Build history of the part. All positions in model axes, mm. A direction names the side the tool comes from. Coordinates: 2 decimals unless noted, no trailing zeros. Loops run counter-clockwise (first coordinate to the right, second up) from the corner with the lowest first, then second, coordinate; pieces in that order, holes last.
(1) Wall check: L1, parallel to Y at x = 0, z = -0.7; L2, parallel to X at y = -41, z = 12; L3, parallel to Y at x = -8.5, z = 7.25. Give the ranges that are in metal, low to high.
(2) Slice it at B-B (x = 0). Give the number of separate pieces and of enclosed holes in the cut face, and give its area (4 significant figures).
(3) Flat gauge pins, fed straight in: P1, Ø2, axis at x = 30.5, z = 4, coming from the +Y side; P2, Ø5, axis at x = -1, y = -35.5, coming from the +Z side; P3, Ø0.5, axis at x = -31, z = 19, coming from the -Y side. Where does each tip first touch, or does it go through?
(4) Slice it at A-A (z = 13). Give the cut face in (x, y).
(5) Tool access for faces 4 (the face through (-27, 16, 6)), 5 (the face through (28, 43.5, 17)), 6 (the face through (-29, 16, 11)): list every direction of +Z, -Z, +X, -X, +Y, -Y with a clear straight run to the whole face (end or side of a thin tool).
(6) Slice it at D-D (x = -9). Give the cut face in (y, z).
(7) Two-plate mould, pull along Y, no slides. Class faces 1 (the face through (31.297, 48.859, 8.633)), 2 (the face through (-32.5, -1, 9)), 3 (the face through (-30, 41.5, 9)): pulls with the +Y half, pulls with the -Y half, needs draft (parallel to the pull), parting line crosses it, or undercut.
from build123d import *

# Parameters (mm, degrees)
SKETCH_1_W            = 65
SKETCH_1_H            = 100
SKETCH_1_W_2          = 63
SKETCH_1_H_2          = 98
EXTRUDE_1_DEPTH       = 18
SKETCH_3_W            = 65
SKETCH_3_H            = 100
EXTRUDE_2_DEPTH       = 1
SKETCH_4_W            = 7.5
SKETCH_4_H            = 7
SKETCH_4_H_2          = 8
EXTRUDE_3_DEPTH       = 11
SKETCH_8_W            = 7.5
SKETCH_8_H            = 7.5
EXTRUDE_4_DEPTH       = 18
EXTRUDE_10_DEPTH      = 1.5
EXTRUDE_10_DEPTH_BACK = 1.5
SKETCH_17_W           = 48
SKETCH_17_H           = 1
SKETCH_17_W_2         = 1
SKETCH_17_H_2         = 83
SKETCH_11_R           = 3
CUT_EXTRUDE_2_DEPTH   = 18
HOLE_WIZARD_M31_D     = 3.4
SKETCH_5_R            = 1.3
CUT_EXTRUDE_4_DEPTH   = 5
SKETCH_15_W           = 4
SKETCH_15_H           = 10
CUT_EXTRUDE_3_DEPTH   = 1
FILLET_5_R            = 1.5
FILLET_6_R            = 3.5
FILLET_7_R            = 4
SKETCH_16_R           = 6
SKETCH_16_R_2         = 5
EXTRUDE_6_DEPTH       = 2
SKETCH_10_6_R         = 3
SKETCH_10_6_R_2       = 2.5
EXTRUDE_8_DEPTH       = 5
SKETCH_9_4_R          = 4
SKETCH_9_4_R_2        = 2.5
SKETCH_9_4_R_3        = 3
CUT_EXTRUDE_6_DEPTH   = 63.741533293
FILLET_8_R            = 4


with BuildPart() as part:
    # Эскиз1 → Бобышка-Вытянуть1 (new body)
    with BuildSketch(Plane.XY):
        Rectangle(SKETCH_1_W, SKETCH_1_H)
        Rectangle(SKETCH_1_W_2, SKETCH_1_H_2, mode=Mode.SUBTRACT)
    extrude(amount=EXTRUDE_1_DEPTH)

    # Эскиз3 → Бобышка-Вытянуть2 (add)
    with BuildSketch(Plane(origin=(0, 0, 0), x_dir=(-1, 0, 0), z_dir=(0, 0, -1))):
        Rectangle(SKETCH_3_W, SKETCH_3_H)
    extrude(amount=EXTRUDE_2_DEPTH)

    # Эскиз4 → Бобышка-Вытянуть3 (add)
    with BuildSketch(Plane.XY):
        with Locations((-27.75, 16)):
            Rectangle(SKETCH_4_W, SKETCH_4_H)
        with Locations((27.75, 16)):
            Rectangle(SKETCH_4_W, SKETCH_4_H)
        with Locations((-27.75, -37.5)):
            Rectangle(SKETCH_4_W, SKETCH_4_H_2)
        with Locations((27.75, -37.5)):
            Rectangle(SKETCH_4_W, SKETCH_4_H_2)
    extrude(amount=EXTRUDE_3_DEPTH)

    # Эскиз8 → Бобышка-Вытянуть4 (add)
    with BuildSketch(Plane.XY):
        with Locations((-27.75, 45.25)):
            Rectangle(SKETCH_8_W, SKETCH_8_H)
        with Locations((27.75, 45.25)):
            Rectangle(SKETCH_8_W, SKETCH_8_H)
        with Locations((27.75, -45.25)):
            Rectangle(SKETCH_8_W, SKETCH_8_H)
        with Locations((-27.75, -45.25)):
            Rectangle(SKETCH_8_W, SKETCH_8_H)
    extrude(amount=EXTRUDE_4_DEPTH)

    # Эскиз17 → Бобышка-Вытянуть10 (add, two sides: drawn at the far end of the back side and taken through both)
    with BuildSketch(Plane.XY.offset(18).offset(-EXTRUDE_10_DEPTH_BACK)):
        with Locations((0, 48.5)):
            Rectangle(SKETCH_17_W, SKETCH_17_H)
        with Locations((31, 0)):
            Rectangle(SKETCH_17_W_2, SKETCH_17_H_2)
        with Locations((-31, 0)):
            Rectangle(SKETCH_17_W_2, SKETCH_17_H_2)
        with Locations((0, -48.5)):
            Rectangle(SKETCH_17_W, SKETCH_17_H)
    extrude(amount=EXTRUDE_10_DEPTH + EXTRUDE_10_DEPTH_BACK)

    # Эскиз11 → Вырез-Вытянуть2 (cut)
    with BuildSketch(Plane(origin=(0, 0, -1), x_dir=(-1, 0, 0), z_dir=(0, 0, -1))):
        with Locations((-28, 45.5)):
            Circle(SKETCH_11_R)
        with Locations((28, 45.5)):
            Circle(SKETCH_11_R)
        with Locations((28, -45.5)):
            Circle(SKETCH_11_R)
        with Locations((-28, -45.5)):
            Circle(SKETCH_11_R)
    extrude(amount=-CUT_EXTRUDE_2_DEPTH, mode=Mode.SUBTRACT)

    # Отверстие с зазором M31 (through all)
    with Locations(Plane(origin=(0, 0, 17), x_dir=(-1, 0, 0), z_dir=(0, 0, -1))):
        with Locations((-28, 45.5), (28, 45.5), (28, -45.5), (-28, -45.5)):
            Hole(HOLE_WIZARD_M31_D / 2)

    # Эскиз5 → Вырез-Вытянуть4 (cut)
    with BuildSketch(Plane.XY.offset(11)):
        with Locations((-27, 16)):
            Circle(SKETCH_5_R)
        with Locations((27, 16)):
            Circle(SKETCH_5_R)
        with Locations((-27, -37)):
            Circle(SKETCH_5_R)
        with Locations((27, -37)):
            Circle(SKETCH_5_R)
    extrude(amount=-CUT_EXTRUDE_4_DEPTH, mode=Mode.SUBTRACT)

    # Эскиз15 → Вырез-Вытянуть3 (cut)
    with BuildSketch(Plane.ZY.offset(31.5)):
        with Locations((9.4, -23.5)):
            Rectangle(SKETCH_15_W, SKETCH_15_H)
    extrude(amount=CUT_EXTRUDE_3_DEPTH, mode=Mode.SUBTRACT)

    # Скругление5
    fillet_5_edges = [part.edges().sort_by_distance(p)[0] for p in [
        (-32, -18.5, 11.4),
        (-32, -28.5, 11.4),
        (-32, -28.5, 7.4),
        (-32, -18.5, 7.4),
    ]]
    fillet(fillet_5_edges, radius=FILLET_5_R)

    # Скругление6
    fillet_6_edges = [part.edges().sort_by_distance(p)[0] for p in [
        (-24, 12.5, 5.5),
        (-24, 19.5, 5.5),
        (24, 19.5, 5.5),
        (24, 12.5, 5.5),
        (-24, -33.5, 5.5),
        (24, -33.5, 5.5),
    ]]
    fillet(fillet_6_edges, radius=FILLET_6_R - 0.0001)  # a hair under: the kernel refuses the full size

    # Скругление7
    fillet_7_edges = [part.edges().sort_by_distance(p)[0] for p in [
        (-24, 41.5, 9),
        (24, 41.5, 9),
        (24, -41.5, 14.5),
        (-24, -41.5, 14.5),
    ]]
    fillet(fillet_7_edges, radius=FILLET_7_R)

    # Эскиз16 → Бобышка-Вытянуть6 (add)
    with BuildSketch(Plane.XY):
        with Locations(Location((0, -33, 0), (0, 0, 180))):
            Circle(SKETCH_16_R)
        with Locations((0, -33)):
            Circle(SKETCH_16_R_2, mode=Mode.SUBTRACT)
    extrude(amount=EXTRUDE_6_DEPTH)

    # Эскиз10<6> → Бобышка-Вытянуть8 (add)
    # profile 1 of 3: a face of its own
    with BuildSketch(Plane.XY):
        with BuildLine():
            ThreePointArc((-3.992179856, -14.75), (0, -18.5), (3.992179856, -14.75))
            ThreePointArc((3.992179856, -14.75), (3.998044486, -14.62506114), (4, -14.5))
            ThreePointArc((4, -14.5), (-0.12506114, -10.501955514), (-3.992179856, -14.75))
        make_face()
        with Locations((0, -14.5)):
            Circle(SKETCH_10_6_R, mode=Mode.SUBTRACT)
    # profile 2 of 3: a face of its own
    with BuildSketch(Plane.XY):
        with BuildLine():
            Line((3.493157374, -22.71875), (3.992179856, -14.75))
            ThreePointArc((3.992179856, -14.75), (0, -18.5), (-3.992179856, -14.75))
            Line((-3.992179856, -14.75), (-3.493157374, -22.71875))
            ThreePointArc((-3.493157374, -22.71875), (-0.109428497, -19.001711075), (3.5, -22.5))
            ThreePointArc((3.5, -22.5), (3.498288925, -22.609428497), (3.493157374, -22.71875))
        make_face()
    # profile 3 of 3: a face of its own
    with BuildSketch(Plane.XY):
        with BuildLine():
            ThreePointArc((-3.493157374, -22.71875), (0, -26), (3.493157374, -22.71875))
            ThreePointArc((3.493157374, -22.71875), (3.498288925, -22.609428497), (3.5, -22.5))
            ThreePointArc((3.5, -22.5), (-0.109428497, -19.001711075), (-3.493157374, -22.71875))
        make_face()
        with Locations((0, -22.5)):
            Circle(SKETCH_10_6_R_2, mode=Mode.SUBTRACT)
    extrude(amount=EXTRUDE_8_DEPTH)

    # Эскиз9<4> → Вырез-Вытянуть6 (cut, through all)
    with BuildSketch(Plane.XY):
        with Locations((0, -33)):
            Circle(SKETCH_9_4_R)
        with Locations((0, -22.5)):
            Circle(SKETCH_9_4_R_2)
        with Locations((0, -14.5)):
            Circle(SKETCH_9_4_R_3)
    extrude(amount=-CUT_EXTRUDE_6_DEPTH, mode=Mode.SUBTRACT)

    # Скругление8
    fillet_8_edges = [part.edges().sort_by_distance(p)[0] for p in [
        (32.5, -50, 8.5),
        (-32.5, -50, 8.5),
        (-32.5, 50, 8.5),
        (32.5, 50, 8.5),
    ]]
    fillet(fillet_8_edges, radius=FILLET_8_R)


solid = part.part
Response values:
1. L1: y = -50 to -37, -29 to -25, -20 to -17.5, -11.5 to 50
1. L2: x = -32.5 to -31.5, 31.5 to 32.5
1. L3: y = -50 to -49, 49 to 50
2. separate pieces: 4
2. enclosed holes: 0
2. area: 149.5 mm2
3. P1: stops at y = 49.87
3. P2: stops at z = 2
3. P3: stops at y = -41.5
4. outline: (-32.5, -46) arc R4 ccw to (-28.5, -50) - (28.5, -50) arc R4 ccw to (32.5, -46) - (32.5, 46) arc R4 ccw to (28.5, 50) - (-28.5, 50) arc R4 ccw to (-32.5, 46) - close; hole (-31.5, -41.5) - (-28, -41.5) arc R4 cw to (-24, -45.5) - (-24, -49) - (24, -49) - (24, -45.5) arc R4 cw to (28, -41.5) - (31.5, -41.5) - (31.5, 41.5) - (28, 41.5) arc R4 cw to (24, 45.5) - (24, 49) - (-24, 49) - (-24, 45.5) arc R4 cw to (-28, 41.5) - (-31.5, 41.5) - close; hole circle Ø6 at (-28, -45.5); hole circle Ø6 at (-28, 45.5); hole circle Ø6 at (28, -45.5); hole circle Ø6 at (28, 45.5)
5. face 4: +Z
5. face 5: -Z
5. face 6: none
6. outline: (-50, -1) - (50, -1) - (50, 18) - (49, 18) - (49, 19.5) - (48, 19.5) - (48, 16.5) - (49, 16.5) - (49, 0) - (-49, 0) - (-49, 16.5) - (-48, 16.5) - (-48, 19.5) - (-49, 19.5) - (-49, 18) - (-50, 18) - close
7. face 1: pulls with the +Y half
7. face 2: needs draft
7. face 3: undercut
